Read the model definition and answer for the solid it produces. Units are mm, in the model's axes. A direction names the side the tool comes from. Coordinates: 2 decimals unless noted, no trailing zeros. Use a Markdown table: item, result. Add a question column.
1) For faces 1 (the face through (-793, -25.4, 17)), 2 (the face through (-318, -50.8, 9)), determine the directions among +Z, -Z, +X, -X, +Y, -Y from which every point of the face is accessible in a straight line to the end or side of a thin tool.
2) The mould has two halves that part along X. Classify faces 3 (the face through (-630, 1, 9.525)), 4 (the face through (736, 1, 34.925)), 5 (the face through (852.488, -1, 17)): released by +X, released by -X, zero draft, split by the parting line, or undercut.
3) Find section A-A on z = 19.5. Count the separate pieces of the cut face and the enclosed holes in it, plus the area to 3 significant figures.
4) Find the intervals of material crossed by probe 1 along X at (y, z) = (-37, 6); probe 2 along Y at (x, z) = (-175.5, 13.5); probe 3 along Y at (x, z) = (-770, 5), in increasing order. Write a range as [from, to].
5) Each of these flat-tipped pins is pushed along its axis until it touches: pin 1 Ø19 at (x, y) = (177.5, 11.5) entering from +Z (3 decimals); pin 2 Ø12 at (x, y) = (-623, 14) entering from -Z. Where does it stop, or does it pass through?
from build123d import *

# Parameters (mm, degrees)
SKETCH1_W           = 1704.975
SKETCH1_H           = 101.6
BOSS_EXTRUDE1_DEPTH = 34.925
CUT_EXTRUDE1_DEPTH  = 25.4
SKETCH3_W           = 85.725
SKETCH3_H           = 25.4
CUT_EXTRUDE2_DEPTH  = 855.713597225


with BuildPart() as part:
    # Sketch1 → Boss-Extrude1 (new body)
    with BuildSketch(Plane.XY):
        Rectangle(SKETCH1_W, SKETCH1_H)
    extrude(amount=BOSS_EXTRUDE1_DEPTH)

    # Sketch2 → Cut-Extrude1 (cut)
    with BuildSketch(Plane.XY.offset(34.925)):
        with BuildLine():
            Line((782.26454982, -50.8), (785.8125, 50.8))
            Line((785.8125, 50.8), (820.7375, 50.8))
            Line((820.7375, 50.8), (819.621026714, 18.828388196))
            ThreePointArc((819.621026714, 18.828388196), (817.685975615, 14.482192268), (813.274894962, 12.7))
            Line((813.274894962, 12.7), (813.057018682, 12.7))
            Line((813.057018682, 12.7), (810.83954982, -50.8))
            Line((810.83954982, -50.8), (782.26454982, -50.8))
        make_face()
        with BuildLine():
            Line((658.43954982, -50.8), (661.9875, 50.8))
            Line((661.9875, 50.8), (696.9125, 50.8))
            Line((696.9125, 50.8), (695.796026714, 18.828388196))
            ThreePointArc((695.796026714, 18.828388196), (693.860975615, 14.482192268), (689.449894962, 12.7))
            Line((689.449894962, 12.7), (689.232018682, 12.7))
            Line((689.232018682, 12.7), (687.01454982, -50.8))
            Line((687.01454982, -50.8), (658.43954982, -50.8))
        make_face()
        with BuildLine():
            Line((534.61454982, -50.8), (538.1625, 50.8))
            Line((538.1625, 50.8), (573.0875, 50.8))
            Line((573.0875, 50.8), (571.971026714, 18.828388196))
            ThreePointArc((571.971026714, 18.828388196), (570.035975615, 14.482192268), (565.624894962, 12.7))
            Line((565.624894962, 12.7), (565.407018682, 12.7))
            Line((565.407018682, 12.7), (563.18954982, -50.8))
            Line((563.18954982, -50.8), (534.61454982, -50.8))
        make_face()
        with BuildLine():
            Line((410.78954982, -50.8), (414.3375, 50.8))
            Line((414.3375, 50.8), (449.2625, 50.8))
            Line((449.2625, 50.8), (448.146026714, 18.828388196))
            ThreePointArc((448.146026714, 18.828388196), (446.210975615, 14.482192268), (441.799894962, 12.7))
            Line((441.799894962, 12.7), (441.582018682, 12.7))
            Line((441.582018682, 12.7), (439.36454982, -50.8))
            Line((439.36454982, -50.8), (410.78954982, -50.8))
        make_face()
        with BuildLine():
            Line((286.96454982, -50.8), (290.5125, 50.8))
            Line((290.5125, 50.8), (325.4375, 50.8))
            Line((325.4375, 50.8), (324.321026714, 18.828388196))
            ThreePointArc((324.321026714, 18.828388196), (322.385975615, 14.482192268), (317.974894962, 12.7))
            Line((317.974894962, 12.7), (317.757018682, 12.7))
            Line((317.757018682, 12.7), (315.53954982, -50.8))
            Line((315.53954982, -50.8), (286.96454982, -50.8))
        make_face()
        with BuildLine():
            Line((163.13954982, -50.8), (166.6875, 50.8))
            Line((166.6875, 50.8), (201.6125, 50.8))
            Line((201.6125, 50.8), (200.496026714, 18.828388196))
            ThreePointArc((200.496026714, 18.828388196), (198.560975615, 14.482192268), (194.149894962, 12.7))
            Line((194.149894962, 12.7), (193.932018682, 12.7))
            Line((193.932018682, 12.7), (191.71454982, -50.8))
            Line((191.71454982, -50.8), (163.13954982, -50.8))
        make_face()
        with BuildLine():
            Line((39.31454982, -50.8), (42.8625, 50.8))
            Line((42.8625, 50.8), (77.7875, 50.8))
            Line((77.7875, 50.8), (76.671026714, 18.828388196))
            ThreePointArc((76.671026714, 18.828388196), (74.735975615, 14.482192268), (70.324894962, 12.7))
            Line((70.324894962, 12.7), (70.107018682, 12.7))
            Line((70.107018682, 12.7), (67.88954982, -50.8))
            Line((67.88954982, -50.8), (39.31454982, -50.8))
        make_face()
        with BuildLine():
            Line((-84.51045018, -50.8), (-80.9625, 50.8))
            Line((-80.9625, 50.8), (-46.0375, 50.8))
            Line((-46.0375, 50.8), (-47.153973286, 18.828388196))
            ThreePointArc((-47.153973286, 18.828388196), (-49.089024385, 14.482192268), (-53.500105038, 12.7))
            Line((-53.500105038, 12.7), (-53.717981318, 12.7))
            Line((-53.717981318, 12.7), (-55.93545018, -50.8))
            Line((-55.93545018, -50.8), (-84.51045018, -50.8))
        make_face()
        with BuildLine():
            Line((-208.33545018, -50.8), (-204.7875, 50.8))
            Line((-204.7875, 50.8), (-169.8625, 50.8))
            Line((-169.8625, 50.8), (-170.978973286, 18.828388196))
            ThreePointArc((-170.978973286, 18.828388196), (-172.914024385, 14.482192268), (-177.325105038, 12.7))
            Line((-177.325105038, 12.7), (-177.542981318, 12.7))
            Line((-177.542981318, 12.7), (-179.76045018, -50.8))
            Line((-179.76045018, -50.8), (-208.33545018, -50.8))
        make_face()
        with BuildLine():
            Line((-332.16045018, -50.8), (-328.6125, 50.8))
            Line((-328.6125, 50.8), (-293.6875, 50.8))
            Line((-293.6875, 50.8), (-294.803973286, 18.828388196))
            ThreePointArc((-294.803973286, 18.828388196), (-296.739024385, 14.482192268), (-301.150105038, 12.7))
            Line((-301.150105038, 12.7), (-301.367981318, 12.7))
            Line((-301.367981318, 12.7), (-303.58545018, -50.8))
            Line((-303.58545018, -50.8), (-332.16045018, -50.8))
        make_face()
        with BuildLine():
            Line((-525.83545018, -50.8), (-522.2875, 50.8))
            Line((-522.2875, 50.8), (-487.3625, 50.8))
            Line((-487.3625, 50.8), (-488.478973286, 18.828388196))
            ThreePointArc((-488.478973286, 18.828388196), (-490.414024385, 14.482192268), (-494.825105038, 12.7))
            Line((-494.825105038, 12.7), (-495.042981318, 12.7))
            Line((-495.042981318, 12.7), (-497.26045018, -50.8))
            Line((-497.26045018, -50.8), (-525.83545018, -50.8))
        make_face()
        with BuildLine():
            Line((-649.66045018, -50.8), (-646.1125, 50.8))
            Line((-646.1125, 50.8), (-611.1875, 50.8))
            Line((-611.1875, 50.8), (-612.303973286, 18.828388196))
            ThreePointArc((-612.303973286, 18.828388196), (-614.239024385, 14.482192268), (-618.650105038, 12.7))
            Line((-618.650105038, 12.7), (-618.867981318, 12.7))
            Line((-618.867981318, 12.7), (-621.08545018, -50.8))
            Line((-621.08545018, -50.8), (-649.66045018, -50.8))
        make_face()
        with BuildLine():
            Line((-773.48545018, -50.8), (-769.9375, 50.8))
            Line((-769.9375, 50.8), (-735.0125, 50.8))
            Line((-735.0125, 50.8), (-736.128973286, 18.828388196))
            ThreePointArc((-736.128973286, 18.828388196), (-738.064024385, 14.482192268), (-742.475105038, 12.7))
            Line((-742.475105038, 12.7), (-742.692981318, 12.7))
            Line((-742.692981318, 12.7), (-744.91045018, -50.8))
            Line((-744.91045018, -50.8), (-773.48545018, -50.8))
        make_face()
    extrude(amount=-CUT_EXTRUDE1_DEPTH, mode=Mode.SUBTRACT)

    # Sketch3 → Cut-Extrude2 (cut, through all)
    with BuildSketch(Plane(origin=(0, 0, 0), x_dir=(-1, 0, 0), z_dir=(0, 0, -1))):
        with Locations((784.225, -38.1)):
            Rectangle(SKETCH3_W, SKETCH3_H)
        with Locations((-409.575, -38.1)):
            Rectangle(SKETCH3_W, SKETCH3_H)
    extrude(amount=-CUT_EXTRUDE2_DEPTH, mode=Mode.SUBTRACT)


solid = part.part
Check result:
| question | item | result |
|---|---|---|
| 1 | face 1 | +Z, -Z, -Y |
| 1 | face 2 | +Z, -Z, +X, -X, -Y |
| 2 | face 3 | undercut |
| 2 | face 4 | zero draft |
| 2 | face 5 | released by +X |
| 3 | separate pieces | 14 |
| 3 | enclosed holes | 0 |
| 3 | area | 130,000 mm2 |
| 4 | probe 1 | x = [-852.49, -827.09], [-741.36, 366.71], [452.44, 852.49] |
| 4 | probe 2 | y = [-50.8, 12.97] |
| 4 | probe 3 | y = [-25.4, 50.8] |
| 5 | pin 1 | stops at z = 9.525 |
| 5 | pin 2 | stops at z = 0 |
